Can you work these out from the model? Positions are in its coordinate system, mm. Face numbers are marked on the shaded views. A direction names the side the tool comes from. Give positions to 0.01 mm unless a question says otherwise; leave off trailing zeros. Write each loop counter-clockwise with the first axis right and the second up, starting at its lowest first coordinate (ties: lowest second). Pieces come first, ordered by that corner, then holes. Notation, with made-up numbers: (-6.75, 62.5) -> (-2.75, 62.5) arc R16 ccw to (-2.75, 88.5) -> close; hole circle Ø11 at (-33, 15). An arc over 180 degrees is marked (long way). Answer as CSV lines item,"result". Start each with the question number.
1. I need wall thicknesses on line 1 (Y direction, x = 0, z = -48.05); line 2 (Z direction, x = -5, y = 36.5); line 3 (Y direction, x = 0, z = -47). Which ranges of each line are inside material? Lowest first, please. Write a range as [from, to].
2. On a 3-axis mill with a long thin cutter (end or side, diameter ignored), from which of +Z, -Z, +X, -X, +Y, -Y can I reach the whole of each face in a straight line? I mean the marked faces 4 and 5. Say none if no direction works.
3. If we section it at C-C on z = -27: Write out the boundary of the cut face in (x, y), plus the area to 3 significant figures.
4. If we mould it in two halves opening along Z, with no side actions, what happens to the marked faces 1, 2 and 3? For each: pulls with the +Z half, pulls with the -Z half, needs draft (parallel to the pull), parting line crosses it, or undercut.
5. If we section it at A-A on y = 21: Write out the boundary of the cut face in (x, z), plus the area to 3 significant figures.
6. If we section it at B-B on x = 0: Count the separate pieces of the cut face and the enclosed holes in it, plus the area to 3 significant figures.
7. I'm going to push flat-ended pins straight in: P1, Ø5, axis at x = 0, y = 33, coming from the +Z side; P2, Ø3.5, axis at x = 0, y = 21, coming from the +Z side; P3, Ø8, axis at x = 0.5, z = -26.5, coming from the +Y side; P4, Ø1.5, axis at x = -7, z = -45, coming from the +Y side. Where does each tip first touch, or does it pass through?
```python
from build123d import *

# Parameters (mm, degrees)
SKETCH1_R           = 2
BOSS_EXTRUDE1_DEPTH = 2.5
BOSS_EXTRUDE2_START = -5
SKETCH2_W           = 40
SKETCH2_H           = 5
BOSS_EXTRUDE2_DEPTH = 53
SKETCH3_R           = 2
BOSS_EXTRUDE3_DEPTH = 5
FILLET2_R           = 8
FILLET1_R           = 2
CHAMFER1_SIZE       = 1


with BuildPart() as part:
    # Sketch1 → Boss-Extrude1 (new, symmetric)
    with BuildSketch(Plane.XY):
        with BuildLine():
            Line((-20, 0), (20, 0))
            Line((20, 0), (20, 33))
            ThreePointArc((20, 33), (0, 53), (-20, 33))
            Line((-20, 33), (-20, 0))
        make_face()
        with Locations((0, 33)):
            Circle(SKETCH1_R, mode=Mode.SUBTRACT)
        with Locations((0, 21)):
            Circle(SKETCH1_R, mode=Mode.SUBTRACT)
    extrude(amount=BOSS_EXTRUDE1_DEPTH, both=True)

    # Sketch2 → Boss-Extrude2 (add)
    with BuildSketch(Plane(origin=(0, 0, -2.5), x_dir=(-1, 0, 0), z_dir=(0, 0, -1)).offset(BOSS_EXTRUDE2_START)):
        with Locations((0, 2.5)):
            Rectangle(SKETCH2_W, SKETCH2_H)
    extrude(amount=BOSS_EXTRUDE2_DEPTH)

    # Sketch3 → Boss-Extrude3 (add)
    with BuildSketch(Plane(origin=(0, 0, -50.5), x_dir=(-1, 0, 0), z_dir=(0, 0, -1))):
        with BuildLine():
            Line((-20, 33), (-20, 5))
            Line((-20, 5), (20, 5))
            Line((20, 5), (20, 33))
            ThreePointArc((20, 33), (0, 53), (-20, 33))
        make_face()
        with Locations(Location((0, 21, 0), (0, 0, 180))):
            Circle(SKETCH3_R, mode=Mode.SUBTRACT)
        with Locations(Location((0, 33, 0), (0, 0, 180))):
            Circle(SKETCH3_R, mode=Mode.SUBTRACT)
    extrude(amount=-BOSS_EXTRUDE3_DEPTH)

    # Fillet2
    fillet2_edges = [part.edges().sort_by_distance(p)[0] for p in [
        (0, 5, -2.5),
        (0, 5, -45.5),
    ]]
    fillet(fillet2_edges, radius=FILLET2_R)

    # Fillet1
    fillet1_edges = [part.edges().sort_by_distance(p)[0] for p in [
        (0, 53, -45.5),
        (20, 23, -45.5),
        (-20, 23, -2.5),
        (-20, 5, -24),
        (20, 5, -24),
        (0, 53, -2.5),
        (-20, 23, -45.5),
        (20, 23, -2.5),
        (-20, 7.343145751, -43.156854249),
        (20, 7.343145751, -43.156854249),
        (-20, 7.343145751, -4.843145751),
        (20, 7.343145751, -4.843145751),
    ]]
    fillet(fillet1_edges, radius=FILLET1_R)

    # Chamfer1
    chamfer1_edges = [part.edges().sort_by_distance(p)[0] for p in [
        (-2, 33, -2.5),
        (-2, 33, 2.5),
        (-2, 21, -2.5),
        (-2, 21, 2.5),
        (-2, 33, -45.5),
        (-2, 21, -45.5),
        (-2, 21, -50.5),
        (-2, 33, -50.5),
    ]]
    chamfer(chamfer1_edges, length=CHAMFER1_SIZE)


solid = part.part
```
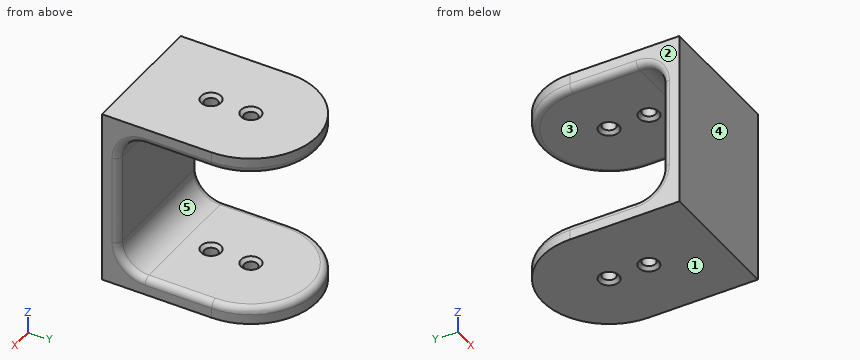
Computed values:
1,line 1,"y = [0, 19], [23, 31], [35, 53]"
1,line 2,"z = [-50.5, -45.5], [-2.5, 2.5]"
1,line 3,"y = [0, 19], [23, 31], [35, 52.94]"
2,face 4,"+Z, -Z, +X, -X, -Y"
2,face 5,"+X, -X, +Y"
3,outline,"(-20, 0) -> (20, 0) -> (20, 3) arc R2 ccw to (18, 5) -> (-18, 5) arc R2 ccw to (-20, 3) -> close"
3,area,"198 mm2"
4,face 1,"pulls with the -Z half"
4,face 2,"needs draft"
4,face 3,"undercut"
5,outline,"(-20, -50.5) -> (-3, -50.5) -> (-2, -49.5) -> (-2, -46.5) -> (-3, -45.5) -> (-18, -45.5) arc R2 ccw to (-20, -47.5) -> close; (-20, -0.5) arc R2 ccw to (-18, -2.5) -> (-3, -2.5) -> (-2, -1.5) -> (-2, 1.5) -> (-3, 2.5) -> (-20, 2.5) -> close; (2, -49.5) -> (3, -50.5) -> (20, -50.5) -> (20, -47.5) arc R2 ccw to (18, -45.5) -> (3, -45.5) -> (2, -46.5) -> close; (2, -1.5) -> (3, -2.5) -> (18, -2.5) arc R2 ccw to (20, -0.5) -> (20, 2.5) -> (3, 2.5) -> (2, 1.5) -> close"
5,area,"353 mm2"
6,separate pieces,"5"
6,enclosed holes,"0"
6,area,"683 mm2"
7,P1,"stops at z = 2"
7,P2,"passes through"
7,P3,"stops at y = 5"
7,P4,"stops at y = 50.66"
